Read the model definition and answer for the solid it produces. Units are mm, in the model's axes. A direction names the side the tool comes from. Round coordinates to 2 decimals unless told otherwise and drop trailing zeros. Order: outer loops, then holes, each group sorted by start corner. A loop starts at its lowest first (then second) coordinate and runs counter-clockwise, first axis right, second up. Notation, with made-up numbers: (-24.75, 55.5) -> (30.25, 55.5) arc R26 ccw to (30.25, 88.5) -> close; hole circle Ø6 at (83, 58.5). An arc over 180 degrees is marked (long way). One line per item, written item: value. Start each with the question number.
1. Consider line 1 (X direction, y = 10.5, z = 0); line 2 (Y direction, x = 2, z = -1.4). Determine where each line is inside the solid, lowest interval first.
2. For faces 1 (the face through (0, -23, -2)), 2 (the face through (0.1, 18.6, 2.5)), determine the directions among +Z, -Z, +X, -X, +Y, -Y from which every point of the face is accessible in a straight line to the end or side of a thin tool.
3. Section A-A (x = 0) is taken. Give the vertices of the cut face in (y, z), then the cut area to 3 significant figures.
4. Flat-ended cylindrical pins translate along their axes: pin 1 Ø1.5 at (x, y) = (0, -23) entering from -Z; pin 2 Ø1 at (y, z) = (19, 1) entering from -X; pin 3 Ø3 at (x, y) = (-0.5, 19) entering from -Z; pin 4 Ø1 at (y, z) = (-16.5, 2) entering from -X. Find the tip coordinate at first contact, or state that the pin passes through.
5. The mould has two halves that part along Y. Classify faces 3 (the face through (0, 27, 0)), 4 (the face through (0, -27, 0)), 5 (the face through (1.29, 10.604, -2.024)): released by +Y, released by -Y, zero draft, split by the parting line, or undercut.
6. Section B-B (y = 0) is taken. Give the vertices of the cut face in (x, z), then the cut area to 3 significant figures.
from build123d import *

# Parameters (mm, degrees)
SKETCH1_R           = 2.5
BOSS_EXTRUDE1_DEPTH = 27
CUT_EXTRUDE2_START  = -9.5
CUT_EXTRUDE2_DEPTH  = 2.5
CUT_EXTRUDE3_START  = -52.5
CUT_EXTRUDE3_DEPTH  = 6
FILLET1_R           = 0.5
SKETCH5_W           = 2
SKETCH5_H           = 0.6


with BuildPart() as part:
    # Sketch1 → Boss-Extrude1 (new, symmetric)
    with BuildSketch(Plane.XZ):
        with Locations(Location((0, 0, 0), (0, 0, 270))):
            Circle(SKETCH1_R)
    extrude(amount=BOSS_EXTRUDE1_DEPTH, both=True)

    # Sketch4 → Cut-Extrude2 (cut)
    with BuildSketch(Plane(origin=(0, 27, 0), x_dir=(1, 0, 0), z_dir=(0, 1, 0)).offset(CUT_EXTRUDE2_START)):
        with BuildLine():
            Line((-1.5, 2), (1.5, 2))
            ThreePointArc((1.5, 2), (0, 2.5), (-1.5, 2))
        make_face()
    extrude(amount=CUT_EXTRUDE2_DEPTH, mode=Mode.SUBTRACT)

    # Sketch4_2 → Cut-Extrude3 (cut)
    with BuildSketch(Plane(origin=(0, 27, 0), x_dir=(1, 0, 0), z_dir=(0, 1, 0)).offset(CUT_EXTRUDE3_START)):
        with BuildLine():
            Line((-1.5, 2), (1.5, 2))
            ThreePointArc((1.5, 2), (0, 2.5), (-1.5, 2))
        make_face()
    extrude(amount=CUT_EXTRUDE3_DEPTH, mode=Mode.SUBTRACT)

    # Fillet1
    fillet1_edges = [part.edges().sort_by_distance(p)[0] for p in [
        (0, 27, 2.5),
        (0, -27, 2.5),
    ]]
    fillet(fillet1_edges, radius=FILLET1_R)

    # Sketch5 → Cut-Revolve2 (revolve, cut)
    with BuildSketch(Plane.XY):
        with Locations((3.4, 10.6)):
            Rectangle(SKETCH5_W, SKETCH5_H)
    revolve(axis=Axis((0, 0, 0), (0, 1, 0)), mode=Mode.SUBTRACT)


solid = part.part
Answer:
1. line 1: -2.4 to 2.4
1. line 2: -26.74 to 10.3, 10.9 to 26.74
2. face 1: -Z, +X, -X
2. face 2: +Y, -Y
3. outline: (-27, -2) arc R0.5 ccw to (-26.5, -2.5) -> (-25.5, -2.5) -> (-25.5, -2) -> (-19.5, -2) -> (-19.5, -2.5) -> (10.3, -2.5) -> (10.3, -2.4) -> (10.9, -2.4) -> (10.9, -2.5) -> (17.5, -2.5) -> (17.5, -2) -> (20, -2) -> (20, -2.5) -> (26.5, -2.5) arc R0.5 ccw to (27, -2) -> (27, 2) arc R0.5 ccw to (26.5, 2.5) -> (10.9, 2.5) -> (10.9, 2.4) -> (10.3, 2.4) -> (10.3, 2.5) -> (-26.5, 2.5) arc R0.5 ccw to (-27, 2) -> close
3. area: 265 mm^2
4. pin 1: z = -2
4. pin 2: x = -2.45
4. pin 3: z = -2.5
4. pin 4: x = -2
5. face 3: released by +Y
5. face 4: released by -Y
5. face 5: undercut
6. outline: circle Ø5 at (0, 0)
6. area: 19.6 mm^2
